Source: CAD feature listing. Evaluate the final solid. Frame: model axes, mm. A direction names the side the tool comes from. Coordinates: 2 decimals unless noted, no trailing zeros. Loops run counter-clockwise (first coordinate to the right, second up) from the corner with the lowest first, then second, coordinate; pieces in that order, holes last. Notation, with made-up numbers: (-37, 38) - (-18, 38) arc R22 cw to (-18, 48) - close; hole circle Ø5 at (-21.75, -11). An arc over 180 degrees is marked (long way). Use one line per item in the form item = value. Start each with the question number.
from build123d import *

# Parameters (mm, degrees)
BOSS_EXTRUDE1_DEPTH = 10
CUT_EXTRUDE2_REACH  = 22.75
SKETCH4_R           = 1.25
SKETCH5_R           = 1.25
CUT_EXTRUDE3_DEPTH  = 4
FILLET1_R           = 1.5


with BuildPart() as part:
    # Sketch1 → Boss-Extrude1 (new body)
    with BuildSketch(Plane.XY):
        Polygon((-32.25, 0), (-32.25, -3.15), (-25, -3.15), (-25, -14.75), (25, -14.75), (25, -3.15), (32.25, -3.15), (32.25, 0), (25, 0), (25, 3), (35.25, 3), (35.25, -6.15), (28, -6.15), (28, -17.75), (-28, -17.75), (-28, -6.15), (-35.25, -6.15), (-35.25, 3), (-25, 3), (-25, 0), align=None)
    extrude(amount=BOSS_EXTRUDE1_DEPTH)

    # Sketch4 → Cut-Extrude2 (cut, up to next)
    with BuildSketch(Plane(origin=(0, 3, 0), x_dir=(1, 0, 0), z_dir=(0, 1, 0)), mode=Mode.PRIVATE) as cut_extrude2_sk1:
        with Locations((-28.625, -5)):
            Circle(SKETCH4_R)
    cut_extrude2_tool1 = extrude(cut_extrude2_sk1.sketch, amount=-CUT_EXTRUDE2_REACH, mode=Mode.PRIVATE) & part.part
    add(cut_extrude2_tool1.solids().sort_by_distance((-28.625, 3, 5))[0], mode=Mode.SUBTRACT)
    # Sketch4 → Cut-Extrude2 (cut, up to next)
    with BuildSketch(Plane(origin=(0, 3, 0), x_dir=(1, 0, 0), z_dir=(0, 1, 0)), mode=Mode.PRIVATE) as cut_extrude2_sk2:
        with Locations((28.625, -5)):
            Circle(SKETCH4_R)
    cut_extrude2_tool2 = extrude(cut_extrude2_sk2.sketch, amount=-CUT_EXTRUDE2_REACH, mode=Mode.PRIVATE) & part.part
    add(cut_extrude2_tool2.solids().sort_by_distance((28.625, 3, 5))[0], mode=Mode.SUBTRACT)

    # Sketch5 → Cut-Extrude3 (cut, through all)
    with BuildSketch(Plane(origin=(0, -14.75, 0), x_dir=(1, 0, 0), z_dir=(0, 1, 0))):
        with Locations((0, -5)):
            Circle(SKETCH5_R)
    extrude(amount=-CUT_EXTRUDE3_DEPTH, mode=Mode.SUBTRACT)

    # Fillet1
    fillet1_edges = [part.edges().sort_by_distance(p)[0] for p in [
        (-25, -14.75, 5),
        (25, -14.75, 5),
        (25, 3, 5),
        (35.25, 3, 5),
        (35.25, -6.15, 5),
        (28, -6.15, 5),
        (28, -17.75, 5),
        (-28, -17.75, 5),
        (-28, -6.15, 5),
        (-35.25, -6.15, 5),
        (-35.25, 3, 5),
        (-25, 3, 5),
    ]]
    fillet(fillet1_edges, radius=FILLET1_R)


solid = part.part
(1) Cut plane B-B, the plane z = 5. State how many separate pieces and enclosed holes the cut face has, plus the area to 3 significant figures.
(2) Contact query for flat-ended pins moving along their axis: pin 1 (1.5 mm diameter, centred on x = -28.625, z = 5, fed in from +Y); pin 2 (2 mm diameter, centred on x = -32, z = 7, fed in from -Y); pin 3 (3.5 mm diameter, centred on x = -29, z = 3, fed in from -Y). Output: stop coordinate, or through.
(3) Cut plane A-A, the plane x = 0. Output: boundary loops of the cut face in (y, z).
(4) Cut plane D-D, the plane x = 21. Output: boundary loops of the cut face in (y, z), plus the area to 3 significant figures.
(5) Material intervals for line 1 (X direction, y = 1.6, z = 5) (3 decimals); line 2 (X direction, y = -16.15, z = 5); line 3 (X direction, y = 2.05, z = 5) (3 decimals), sorted ascending.
(6) Access query for faces 4 (the face through (-32, -6.15, 5)), 5 (the face through (-32.25, -2, 5)), 6 (the face through (25, -8, 5)), 7 (the face through (-35.25, -2, 5)). Directions: +Z, -Z, +X, -X, +Y, -Y. A direction counts if a zero-diameter tool reaches every point of the face in a straight line with its end or side. Return the directions, or none.
(7) Mould query, pull axis Z, two halves, no side actions, for faces 1 (the face through (0, -16, 10)), 2 (the face through (29.78, 1.52, 5.48)), 3 (the face through (0, -14.75, 3)). Classes: +Z half, -Z half, draft (parallel to the pull), parting line (faces both ways), or undercut.
Recorded:
q1.separate_pieces = 4
q1.enclosed_holes = 0
q1.area = 337 mm²
q2.pin_1 = -3.15
q2.pin_2 = -6.15
q2.pin_3 = -17.55
q3.outline = (-17.75, 0) - (-14.75, 0) - (-14.75, 3.75) - (-17.75, 3.75) - close; (-17.75, 6.25) - (-14.75, 6.25) - (-14.75, 10) - (-17.75, 10) - close
q4.outline = (-17.75, 0) - (-14.75, 0) - (-14.75, 10) - (-17.75, 10) - close
q4.area = 30.0 mm²
q5.line_1 = -35.247 to -29.875, -27.375 to -25.003, 25.003 to 27.375, 29.875 to 35.247
q5.line_2 = -28 to -1.25, 1.25 to 28
q5.line_3 = -35.146 to -29.875, -27.375 to -25.104, 25.104 to 27.375, 29.875 to 35.146
q6.face_4 = +Z, -Z, -X, -Y
q6.face_5 = +Z, -Z
q6.face_6 = +Z, -Z, +Y
q6.face_7 = +Z, -Z, -X, +Y, -Y
q7.face_1 = +Z half
q7.face_2 = undercut
q7.face_3 = draft
